Source: three-view drawing plus pictorial views. Frame: mm from the lowest corner of the part. Give positions to 0.01 mm unless a question says otherwise; leave off trailing zeros. Loops run counter-clockwise (first coordinate to the right, second up) from the corner with the lowest first, then second, coordinate; pieces in that order, holes last. Notation, with made-up numbers: M -40,19.5 L -5,19.5 A18 cw -5,50.5 Z; hole C 18,78.25 d4. An arc over 180 degrees is marked long. Answer as a JSON object with one key per item and string values. Group by question number.
1) Section query B-B on z = 11.25. Return loops of the section in (x, y) (1 decimal).
2) Ray query, L1, parallel to X at y = 29, z = 14.75 (1 decimal); L2, parallel to Y at x = 35, z = 14; L3, parallel to Z at x = 68.5, y = 35 (1 decimal). Return the intervals inside material, ascending.
3) First-contact query: P1, Ø8, axis at y = 40.5, z = 4.5, coming from the -X side; P2, Ø2.5, axis at x = 35, y = 72.47, coming from the +Z side; P3, Ø6, axis at x = 33.5, z = 10, coming from the -Y side (1 decimal); P4, Ø3, axis at y = 64.5, z = 11.5, coming from the +X side. Flat tips, straight axial feed; report the tip coordinate or a pass-through.
4) Section query A-A on z = 6. Return loops of the section in (x, y) (1 decimal), plus the area to 3 significant figures.
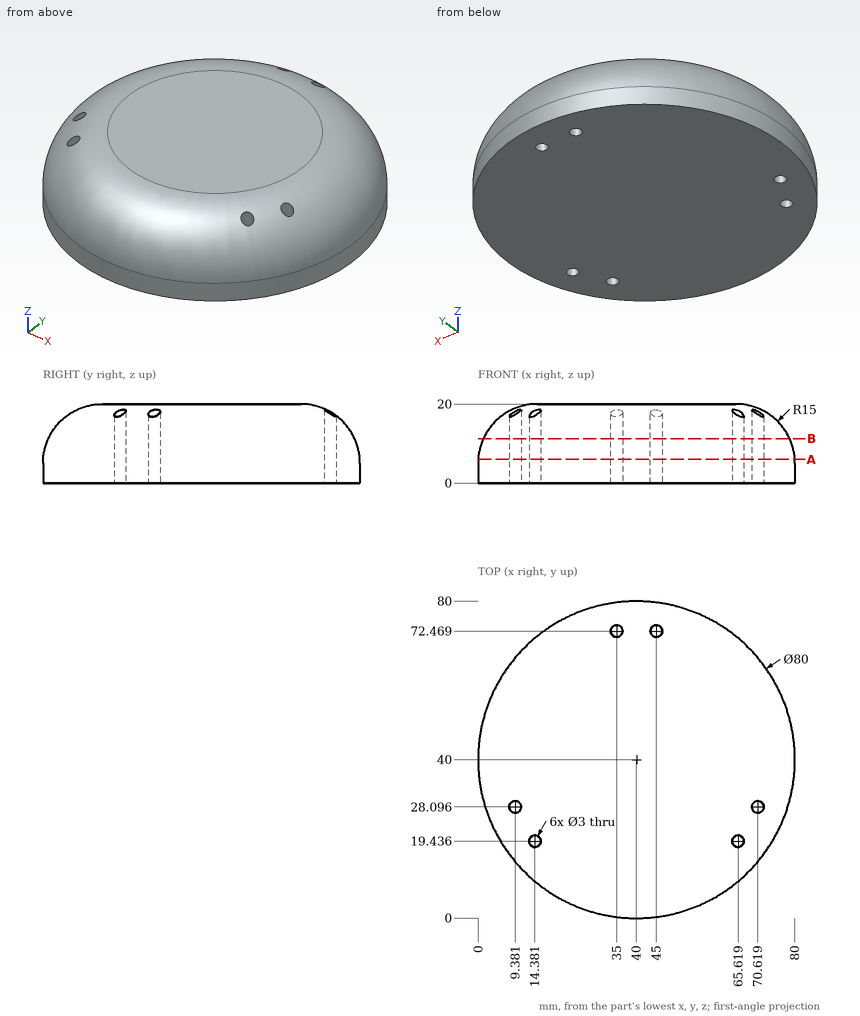
Output:
{
 "1": {"outline": "C 40,40 d77.3; hole C 9.4,28.1 d3; hole C 14.4,19.4 d3; hole C 35,72.5 d3; hole C 45,72.5 d3; hole C 65.6,19.4 d3; hole C 70.6,28.1 d3"},
 "2": {"L1": "x = 5.3 to 8.2, 10.6 to 69.4, 71.8 to 74.7", "L2": "y = 3.34 to 70.97, 73.97 to 76.66", "L3": "z = 0 to 19.5"},
 "3": {"P1": "stops at x = 0", "P2": "passes through", "P3": "stops at y = 0.5", "P4": "stops at x = 71.17"},
 "4": {"outline": "C 40,40 d79.9; hole C 9.4,28.1 d3; hole C 14.4,19.4 d3; hole C 35,72.5 d3; hole C 45,72.5 d3; hole C 65.6,19.4 d3; hole C 70.6,28.1 d3", "area": "4,980 mm^2"}
}
